Input: part model. Units: mm. Frame: model coordinates. A direction names the side the tool comes from. Give positions to 0.01 mm unless a question says otherwise; leave off trailing zeros. Loops run counter-clockwise (first coordinate to the right, second up) from the corner with the lowest first, then second, coordinate; pieces in that order, holes last. Notation, with made-up numbers: (-39, 38) -> (15, 38) arc R30 ccw to (15, 71) -> close; hole circle Ø5 at (-15.5, -25.5). An arc over 180 degrees is marked (long way). Answer as a JSON object with one key per item and string values.
```python
from build123d import *

# Parameters (mm, degrees)
SKETCH1_W           = 63.5
SKETCH1_H           = 63.5
BOSS_EXTRUDE1_DEPTH = 101.6
SKETCH3_W           = 38.1
SKETCH3_H           = 11.43
CUT_EXTRUDE1_DEPTH  = 112.079633597
SKETCH5_R           = 6.35
BOSS_EXTRUDE2_DEPTH = 19.05
SKETCH6_R           = 6.858
CUT_EXTRUDE3_DEPTH  = 19.05


with BuildPart() as part:
    # Sketch1 → Boss-Extrude1 (new body)
    with BuildSketch(Plane(origin=(0, 0, 0), x_dir=(1, 0, 0), z_dir=(0, 1, 0))):
        Rectangle(SKETCH1_W, SKETCH1_H)
    extrude(amount=BOSS_EXTRUDE1_DEPTH)

    # Sketch3 → Cut-Extrude1 (cut, through all)
    with BuildSketch(Plane(origin=(0, 101.6, 0), x_dir=(1, 0, 0), z_dir=(0, 1, 0))):
        Rectangle(SKETCH3_W, SKETCH3_H)
    extrude(amount=-CUT_EXTRUDE1_DEPTH, mode=Mode.SUBTRACT)

    # Sketch5 → Boss-Extrude2 (add)
    with BuildSketch(Plane(origin=(0, 101.6, 0), x_dir=(1, 0, 0), z_dir=(0, 1, 0))):
        with Locations(Location((19.05, -18.7325, 0), (0, 0, 90))):
            Circle(SKETCH5_R)
        with Locations(Location((-19.05, -18.7325, 0), (0, 0, 90))):
            Circle(SKETCH5_R)
        with Locations(Location((-19.05, 18.7325, 0), (0, 0, 90))):
            Circle(SKETCH5_R)
        with Locations(Location((19.05, 18.7325, 0), (0, 0, 90))):
            Circle(SKETCH5_R)
    extrude(amount=BOSS_EXTRUDE2_DEPTH)

    # Sketch6 → Cut-Extrude3 (cut)
    with BuildSketch(Plane.XZ):
        with Locations(Location((18.542, -18.796, 0), (0, 0, 270))):
            Circle(SKETCH6_R)
        with Locations(Location((-18.542, -18.796, 0), (0, 0, 270))):
            Circle(SKETCH6_R)
        with Locations(Location((-18.542, 18.669, 0), (0, 0, 270))):
            Circle(SKETCH6_R)
        with Locations(Location((18.542, 18.669, 0), (0, 0, 270))):
            Circle(SKETCH6_R)
    extrude(amount=-CUT_EXTRUDE3_DEPTH, mode=Mode.SUBTRACT)


solid = part.part
```
Q1. Pin query (flat end, axial travel): pin 1 (1.5 mm diameter, centred on y = 103, z = 17.5, fed in from -X); pin 2 (7 mm diameter, centred on x = 18.5, z = 18, fed in from -Y); pin 3 (6 mm diameter, centred on x = 5, z = -2.5, fed in from -Y). Return the tip coordinate at first contact, or that it passes through.
Evaluation:
{"pin 1": "stops at x = -25.38", "pin 2": "stops at y = 19.05", "pin 3": "passes through"}
Q2. Access query for faces 1 (the cylindrical face through (21.48, 110.99, -24.6)), 2 (the flat face through (-19.05, 52, 0)), 3 (the flat face through (19, 19.05, 19)). Directions: +Z, -Z, +X, -X, +Y, -Y. A direction counts if a zero-diameter tool reaches every point of the face in a straight line with its end or side. Return the directions, or none.
Evaluation:
{"face 1": "+Y", "face 2": "+Y, -Y", "face 3": "-Y"}
Q3. Ray query, line 1 along Z through (x, y) = (-4, 72) (3 decimals); line 2 along X through (y, z) = (77, -2); line 3 along Y through (x, z) = (-22.5, -6). Return the intervals inside material, ascending.
Evaluation:
{"line 1": "z = -31.75 to -5.715, 5.715 to 31.75", "line 2": "x = -31.75 to -19.05, 19.05 to 31.75", "line 3": "y = 0 to 101.6"}
Q4. Section A-A, the plane y = 55.5. Return the cut outline in (x, z) (3 decimals), then the cut area to 3 significant figures.
Evaluation:
{"outline": "(-31.75, -31.75) -> (31.75, -31.75) -> (31.75, 31.75) -> (-31.75, 31.75) -> close; hole (-19.05, -5.715) -> (19.05, -5.715) -> (19.05, 5.715) -> (-19.05, 5.715) -> close", "area": "3,600 mm2"}
Q5. Draft query along Z for faces 4 (the flat face through (0, 50, 31.75)), 5 (the flat face through (0, 52, -5.715)), 6 (the flat face through (19, 120.65, 19)). Return one class per face: +Z half, -Z half, draft (parallel to the pull), parting line (faces both ways), or undercut.
Evaluation:
{"face 4": "+Z half", "face 5": "undercut", "face 6": "draft"}
Q6. Section D-D, the plane z = -7.5. Return the cut outline in (x, y).
Evaluation:
{"outline": "(-31.75, 0) -> (31.75, 0) -> (31.75, 101.6) -> (-31.75, 101.6) -> close"}
Q7. Section B-B, the plane x = -8.5. Return the cut outline in (y, z) (3 decimals).
Evaluation:
{"outline": "(0, -31.75) -> (101.6, -31.75) -> (101.6, -5.715) -> (0, -5.715) -> close; (0, 5.715) -> (101.6, 5.715) -> (101.6, 31.75) -> (0, 31.75) -> close"}
Q8. Section C-C, the plane y = 13. Return the cut outline in (x, z) (3 decimals), then the cut area to 3 significant figures.
Evaluation:
{"outline": "(-31.75, -31.75) -> (31.75, -31.75) -> (31.75, 31.75) -> (-31.75, 31.75) -> close; hole circle Ø13.716 at (-18.542, -18.796); hole circle Ø13.716 at (-18.542, 18.669); hole (-19.05, -5.715) -> (19.05, -5.715) -> (19.05, 5.715) -> (-19.05, 5.715) -> close; hole circle Ø13.716 at (18.542, -18.796); hole circle Ø13.716 at (18.542, 18.669)", "area": "3,010 mm2"}
